from build123d import *

# Parameters (mm, degrees)
F1_DEPTH = 12.7


with BuildPart() as f1:
    # F0 (on Top) → F1 (new body)
    with BuildSketch(Plane.XY):
        with BuildLine():
            Line((-19.05, -12.7), (26.67, -12.7))
            ThreePointArc((26.67, -12.7), (30.262102, -11.212102), (31.75, -7.62))
            Line((31.75, -7.62), (31.75, -1.651))
            Line((31.75, -1.651), (27.691787, -1.651))
            ThreePointArc((27.691787, -1.651), (24.979809, -3.175), (22.267831, -1.651))
            Line((22.267831, -1.651), (-12.918385, -1.651))
            ThreePointArc((-12.918385, -1.651), (-25.4, 0), (-12.918385, 1.651))
            Line((-12.918385, 1.651), (22.267831, 1.651))
            ThreePointArc((22.267831, 1.651), (24.979809, 3.175), (27.691787, 1.651))
            Line((27.691787, 1.651), (31.75, 1.651))
            Line((31.75, 1.651), (31.75, 7.62))
            ThreePointArc((31.75, 7.62), (30.262102, 11.212102), (26.67, 12.7))
            Line((26.67, 12.7), (-19.05, 12.7))
            ThreePointArc((-19.05, 12.7), (-28.030256, 8.980256), (-31.75, 0))
            ThreePointArc((-31.75, 0), (-28.030256, -8.980256), (-19.05, -12.7))
        make_face()
    extrude(amount=F1_DEPTH)


solid = f1.part
Design review of the part built by this model. Coordinates are the model's own, in mm. A direction names the side the tool comes from. Round coordinates to 2 decimals unless told otherwise and drop trailing zeros. Write each loop counter-clockwise with the first axis right and the second up, starting at its lowest first coordinate (ties: lowest second). Pieces come first, ordered by that corner, then holes.
Item 1: Wall thickness on L1, parallel to Y at x = 16, z = 10.5; L2, parallel to Y at x = -19.05, z = 6.5; L3, parallel to X at y = 0, z = 7: over which ranges is each line inside the solid? List them lowest first.
Item 2: Consider section A-A on x = -3. Give the boundary of the cut face in (y, z), and give its area (3 significant figures).
Item 3: Consider section D-D on y = -1. Give the boundary of the cut face in (x, z), and give its area (3 significant figures).
Item 4: Consider section C-C on z = 2. Give the boundary of the cut face in (x, y) (3 decimals), and give its area (3 significant figures).
Item 5: For pin 1 Ø1 at (x, y) = (7.5, -1) entering from +Z; pin 2 Ø3 at (x, y) = (7, 1.5) entering from -Z; pin 3 Ø2 at (x, z) = (29.5, 4.5) entering from +Y; pin 4 Ø2 at (x, z) = (30, 9) entering from -Y, all flat-tipped, find the tip position at first contact; note any pin that passes through.
Item 6: Draft analysis for pull direction X (two halves, no side actions). For faces 4 (the cylindrical face through (24.934, 3.175, 6.261)), 5 (the flat face through (0, -3, 0)), 6 (the cylindrical face through (30.222, -11.251, 6.261)), state which applies: released by +X, released by -X, zero draft, split by the parting line, or undercut.
Item 7: For faces 1 (the flat face through (4, 12.7, 6)), 2 (the cylindrical face through (25.025, -3.175, 6.261)), 3 (the flat face through (4, 1.651, 6)), list the 3-axis set-ups (+Z, -Z, +X, -X, +Y, -Y) from which the entire face can be reached by the end or side of a thin tool; tool diameter is ignored.
Item 8: Consider section B-B on y = -4.25. Give the boundary of the cut face in (x, z).
Check values:
1. L1: y = -12.7 to -1.65, 1.65 to 12.7
1. L2: y = -12.7 to -6.35, 6.35 to 12.7
1. L3: x = -31.75 to -25.4
2. outline: (-12.7, 0) - (-1.65, 0) - (-1.65, 12.7) - (-12.7, 12.7) - close; (1.65, 0) - (12.7, 0) - (12.7, 12.7) - (1.65, 12.7) - close
2. area: 281 mm2
3. outline: (-31.71, 0) - (-25.32, 0) - (-25.32, 12.7) - (-31.71, 12.7) - close
3. area: 81.2 mm2
4. outline: (-19.05, -12.7) - (26.67, -12.7) arc R5.08 ccw to (31.75, -7.62) - (31.75, -1.651) - (27.692, -1.651) arc R3.175 cw to (22.268, -1.651) - (-12.918, -1.651) arc R6.35 cw (long way) to (-12.918, 1.651) - (22.268, 1.651) arc R3.175 cw to (27.692, 1.651) - (31.75, 1.651) - (31.75, 7.62) arc R5.08 ccw to (26.67, 12.7) - (-19.05, 12.7) arc R12.7 ccw to start
4. area: 1,250 mm2
5. pin 1: passes through
5. pin 2: stops at z = 0
5. pin 3: stops at y = 12.36
5. pin 4: stops at y = -12.13
6. face 4: undercut
6. face 5: zero draft
6. face 6: released by +X
7. face 1: +Z, -Z, +X, -X, +Y
7. face 2: +Z, -Z
7. face 3: +Z, -Z, +X
8. outline: (-31.02, 0) - (-23.77, 0) - (-23.77, 12.7) - (-31.02, 12.7) - close; (-14.33, 0) - (31.75, 0) - (31.75, 12.7) - (-14.33, 12.7) - close
